from build123d import *

# Parameters (mm, degrees)
CROQUIS1_W              = 12
CROQUIS1_H              = 22.5
SALIENTE_EXTRUIR1_DEPTH = 22.5
CROQUIS2_W              = 5
CROQUIS2_H              = 2.5
SALIENTE_EXTRUIR2_DEPTH = 12
CROQUIS3_R              = 6
SALIENTE_EXTRUIR3_DEPTH = 4.5
CROQUIS4_R              = 2.4
SALIENTE_EXTRUIR4_DEPTH = 3.1
CROQUIS5_R              = 2.75
SALIENTE_EXTRUIR5_DEPTH = 4.5
REDONDEO1_R             = 2


with BuildPart() as part:
    # Croquis1 → Saliente-Extruir1 (new body)
    with BuildSketch(Plane(origin=(0, 0, 0), x_dir=(1, 0, 0), z_dir=(0, 1, 0))):
        Rectangle(CROQUIS1_W, CROQUIS1_H)
    extrude(amount=SALIENTE_EXTRUIR1_DEPTH)

    # Croquis2 → Saliente-Extruir2 (add)
    with BuildSketch(Plane(origin=(6, 0, 0), x_dir=(0, 0, -1), z_dir=(1, 0, 0))):
        with Locations((-13.75, 17.25)):
            Rectangle(CROQUIS2_W, CROQUIS2_H)
        with Locations((13.75, 17.25)):
            Rectangle(CROQUIS2_W, CROQUIS2_H)
    extrude(amount=-SALIENTE_EXTRUIR2_DEPTH)

    # Croquis3 → Saliente-Extruir3 (add)
    with BuildSketch(Plane(origin=(0, 22.5, 0), x_dir=(1, 0, 0), z_dir=(0, 1, 0))):
        with Locations((0, -5.25)):
            Circle(CROQUIS3_R)
    extrude(amount=SALIENTE_EXTRUIR3_DEPTH)

    # Croquis4 → Saliente-Extruir4 (add)
    with BuildSketch(Plane(origin=(0, 27, 0), x_dir=(1, 0, 0), z_dir=(0, 1, 0))):
        with Locations((0, -5.25)):
            Circle(CROQUIS4_R)
    extrude(amount=SALIENTE_EXTRUIR4_DEPTH)

    # Croquis5 → Saliente-Extruir5 (add)
    with BuildSketch(Plane(origin=(0, 22.5, 0), x_dir=(1, 0, 0), z_dir=(0, 1, 0))):
        with Locations((0, 0.75)):
            Circle(CROQUIS5_R)
    extrude(amount=SALIENTE_EXTRUIR5_DEPTH)

    # Redondeo1
    redondeo1_edges = [part.edges().sort_by_distance(p)[0] for p in [
        (2.676814797, 24.75, -0.119791667),
        (-2.676814797, 24.75, -0.119791667),
    ]]
    fillet(redondeo1_edges, radius=REDONDEO1_R)


solid = part.part
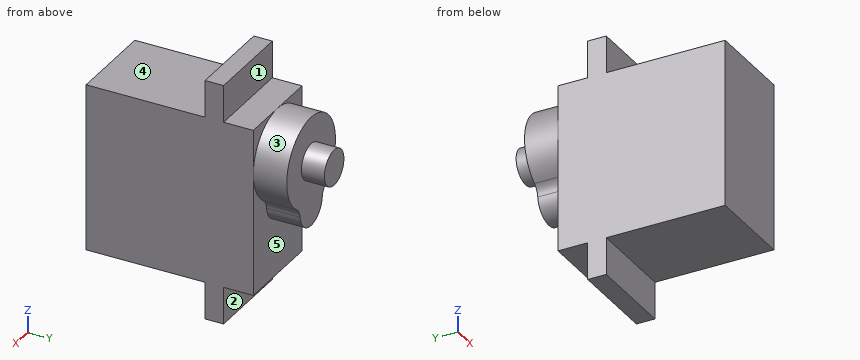
Read the model definition and answer for the solid it produces. Units are mm, in the model's axes. Face numbers are marked on the shaded views. A direction names the side the tool comes from. Give positions to 0.01 mm unless a question says otherwise; leave off trailing zeros. Write each loop counter-clockwise with the first axis right and the second up, starting at its lowest first coordinate (ties: lowest second). Pieces come first, ordered by that corner, then holes. Notation, with made-up numbers: (-9, 62.25) - (8, 62.25) arc R25 ccw to (8, 86.25) - close; hole circle Ø5 at (67, -38.75). An arc over 180 degrees is marked (long way). Answer in a Markdown table with one row per item. Add a question column.
Item 1: Section C-C, the plane z = 10 is taken. Write down the section's boundary in (x, y), and give its area (3 significant figures).
Item 2: Section D-D, the plane x = -4 is taken. Write down the section's boundary in (y, z), and give its area (4 significant figures).
Item 3: A tool of negligible diameter and unlimited length cuts with its end or side. For the marked faces 1, 2, 3, 4 and 5, from which of +Z, -Z, +X, -X, +Y, -Y can it reach the whole face along a straight path? Write none if from no direction.
Item 4: Section B-B, the plane z = -12 is taken. Write down the section's boundary in (x, y), and give its area (3 significant figures).
Item 5: Flat-ended cylindrical pins translate along their axes: P1, Ø3, axis at x = 3.5, z = 8, coming from the +Y side; P2, Ø5, axis at x = 2, y = 11, coming from the -Z side; P3, Ø1.5, axis at x = 3.5, y = 21, coming from the +Z side. Find the tip coordinate at first contact, or state that the pin passes through.
Item 6: Section A-A, the plane x = 1 is taken. Write down the section's boundary in (y, z), and give its area (3 significant figures).
Item 7: Find the intervals of material crossed by L1, parallel to Y at x = 4.5, z = -0.5; L2, parallel to Z at x = -1.25, y = 8; L3, parallel to Y at x = 1.5, z = -14, in increasing order.
Recorded:
| question | item | result |
|---|---|---|
| 1 | outline | (-6, 0) - (6, 0) - (6, 22.5) - (3.67, 22.5) - (3.67, 27) - (-3.67, 27) - (-3.67, 22.5) - (-6, 22.5) - close |
| 1 | area | 303 mm2 |
| 2 | outline | (0, -11.25) - (16, -11.25) - (16, -16.25) - (18.5, -16.25) - (18.5, -11.25) - (22.5, -11.25) - (22.5, 0.78) - (27, 0.78) - (27, 9.72) - (22.5, 9.72) - (22.5, 11.25) - (18.5, 11.25) - (18.5, 16.25) - (16, 16.25) - (16, 11.25) - (0, 11.25) - close |
| 2 | area | 571.5 mm2 |
| 3 | face 1 | +Z, +X, -X, +Y |
| 3 | face 2 | -Z, +X, -X, +Y |
| 3 | face 3 | +Y |
| 3 | face 4 | +Z, +X, -X, -Y |
| 3 | face 5 | -Z, +Y |
| 4 | outline | (-6, 16) - (6, 16) - (6, 18.5) - (-6, 18.5) - close |
| 4 | area | 30.0 mm2 |
| 5 | P1 | stops at y = 27 |
| 5 | P2 | stops at z = -11.25 |
| 5 | P3 | stops at z = 11.25 |
| 6 | outline | (0, -11.25) - (16, -11.25) - (16, -16.25) - (18.5, -16.25) - (18.5, -11.25) - (22.5, -11.25) - (22.5, -3.31) - (27, -3.31) - (27, 3.07) - (30.1, 3.07) - (30.1, 7.43) - (27, 7.43) - (27, 11.17) - (22.5, 11.17) - (22.5, 11.25) - (18.5, 11.25) - (18.5, 16.25) - (16, 16.25) - (16, 11.25) - (0, 11.25) - close |
| 6 | area | 610 mm2 |
| 7 | L1 | y = 0 to 22.5 |
| 7 | L2 | z = -11.25 to 11.25 |
| 7 | L3 | y = 16 to 18.5 |
